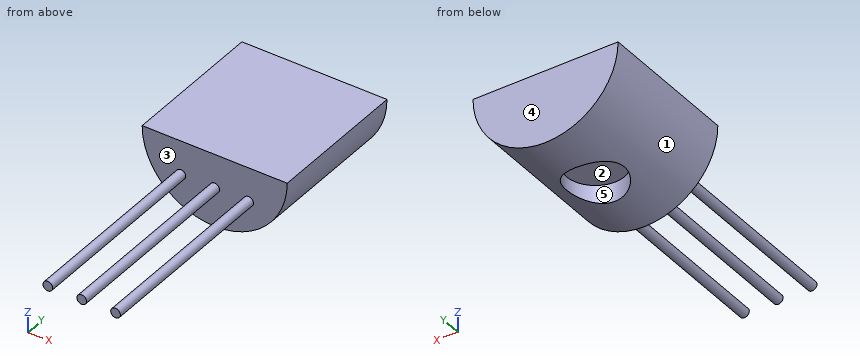
from build123d import *

# Parameters (mm, degrees)
Y_KSEKLIK_EKSTR_ZYON1_DEPTH = 15
IZIM4_R                     = 3
KES_EKSTR_ZYON1_DEPTH       = 2
IZIM8_R                     = 0.5
IZIM10_R                    = 0.5
IZIM11_R                    = 0.5


with BuildPart() as part:
    # Çizim1 → Yükseklik-Ekstrüzyon1 (new body)
    with BuildSketch(Plane(origin=(0, 0, 0), x_dir=(1, 0, 0), z_dir=(0, 1, 0))):
        with BuildLine():
            Line((0, 0), (15, 0))
            ThreePointArc((15, 0), (7.5, 7.5), (0, 0))
        make_face()
    extrude(amount=Y_KSEKLIK_EKSTR_ZYON1_DEPTH)

    # Çizim4 → Kes-Ekstrüzyon1 (cut)
    with BuildSketch(Plane(origin=(7.5, 15, -7.5), x_dir=(-1, 0, 0), z_dir=(0, 0, -1))):
        with Locations((0, -7.5)):
            Circle(IZIM4_R)
    extrude(amount=-KES_EKSTR_ZYON1_DEPTH, mode=Mode.SUBTRACT)

    # Süpür1: sweep along a curve in space
    with BuildLine() as s_p_r1_path:
        Line((11, 0, -3.488617215), (11, -20, -3.488617215))
    # Çizim8 → Süpür1 (sweep)
    with BuildSketch(Plane(origin=(4, -20, -3.488617215), x_dir=(-1, 0, 0), z_dir=(0, -1, 0))):
        with Locations((-7, 0)):
            Circle(IZIM8_R)
    sweep(path=s_p_r1_path.line)

    # Süpür2: sweep along a curve in space
    with BuildLine() as s_p_r2_path:
        Line((7.5, 0, -3.488617215), (7.5, -20, -3.488617215))
    # Çizim10 → Süpür2 (sweep)
    with BuildSketch(Plane(origin=(4, -20, -3.488617215), x_dir=(-1, 0, 0), z_dir=(0, -1, 0))):
        with Locations((-3.5, 0)):
            Circle(IZIM10_R)
    sweep(path=s_p_r2_path.line)

    # Süpür3: sweep along a curve in space
    with BuildLine() as s_p_r3_path:
        Line((4, 0, -3.488617215), (4, -20, -3.488617215))
    # Çizim11 → Süpür3 (sweep)
    with BuildSketch(Plane(origin=(4, -20, -3.488617215), x_dir=(-1, 0, 0), z_dir=(0, -1, 0))):
        Circle(IZIM11_R)
    sweep(path=s_p_r3_path.line)


solid = part.part
Verification items for the finished model (mm, model axes). Face numbers are marked on the shaded views. A direction names the side the tool comes from. Give positions to 0.01 mm unless a question says otherwise; leave off trailing zeros. Loops run counter-clockwise (first coordinate to the right, second up) from the corner with the lowest first, then second, coordinate; pieces in that order, holes last.
1. Cross-section at B-B on y = 7.5. Record the cut outline in (x, z).
Derived:
outline: (0, 0) arc R7.5 ccw to (4.5, -6.87) - (4.5, -5.5) - (10.5, -5.5) - (10.5, -6.87) arc R7.5 ccw to (15, 0) - close
2. Tool access check on the marked faces 1 and 2. Record the directions out of +Z, -Z, +X, -X, +Y, -Y that give a thin tool (end or side, any length) a straight path to the whole face; none if there is none.
Derived:
face 1: -Z, +Y, -Y
face 2: -Z
3. Cross-section at A-A on x = 9. Record the cut outline in (y, z).
Derived:
outline: (0, -7.35) - (4.9, -7.35) - (4.9, -5.5) - (10.1, -5.5) - (10.1, -7.35) - (15, -7.35) - (15, 0) - (0, 0) - close
4. Go/stop test with flat-tipped pins: P1, Ø3, axis at x = 3.5, y = 2, coming from the -Z side; P2, Ø2, axis at x = 5.5, z = -5.5, coming from the -Y side; P3, Ø1.5, axis at x = 12, y = -15, coming from the -Z side. Record where each tip stops, or that it passes through.
Derived:
P1: stops at z = -7.07
P2: stops at y = 0
P3: stops at z = -3.92
5. Cross-section at D-D on y = -2.5. Record the cut outline in (x, z), and give its area (3 significant figures).
Derived:
outline: circle Ø1 at (4, -3.49); circle Ø1 at (7.5, -3.49); circle Ø1 at (11, -3.49)
area: 2.36 mm2
6. Material ranges on probe 1 along Y at (x, z) = (7.5, -6.4); probe 2 along X at (y, z) = (-8, -3.5); probe 3 along Z at (x, y) = (11, -9), recorded low to high.
Derived:
probe 1: y = 0 to 4.5, 10.5 to 15
probe 2: x = 3.5 to 4.5, 7 to 8, 10.5 to 11.5
probe 3: z = -3.99 to -2.99
7. Release check for a two-part mould opening along Y. For the marked faces 3, 4 and 5 record: +Y half, -Y half, draft (parallel to the pull), parting line (faces both ways), or undercut.
Derived:
face 3: -Y half
face 4: +Y half
face 5: undercut
8. Cross-section at C-C on z = -4.5. Record the cut outline in (x, y), and give its area (3 significant figures).
Derived:
outline: (1.5, 0) - (13.5, 0) - (13.5, 15) - (1.5, 15) - close
area: 180 mm2
